Print and shaded views of the part. All mm, measured from the part's lowest x, y and z. A direction names the side the tool comes from. Round coordinates to 2 decimals unless told otherwise and drop trailing zeros. Write each loop counter-clockwise with the first axis right and the second up, starting at its lowest first coordinate (ties: lowest second). Pieces come first, ordered by that corner, then holes. Notation, with made-up numbers: (49, -36.75) -> (64, -36.75) arc R17 cw to (64, -7.75) -> close; hole circle Ø11 at (2.5, 11). An arc over 180 degrees is marked (long way). Return JSON: item names as keys, results as strings. Group by question number.
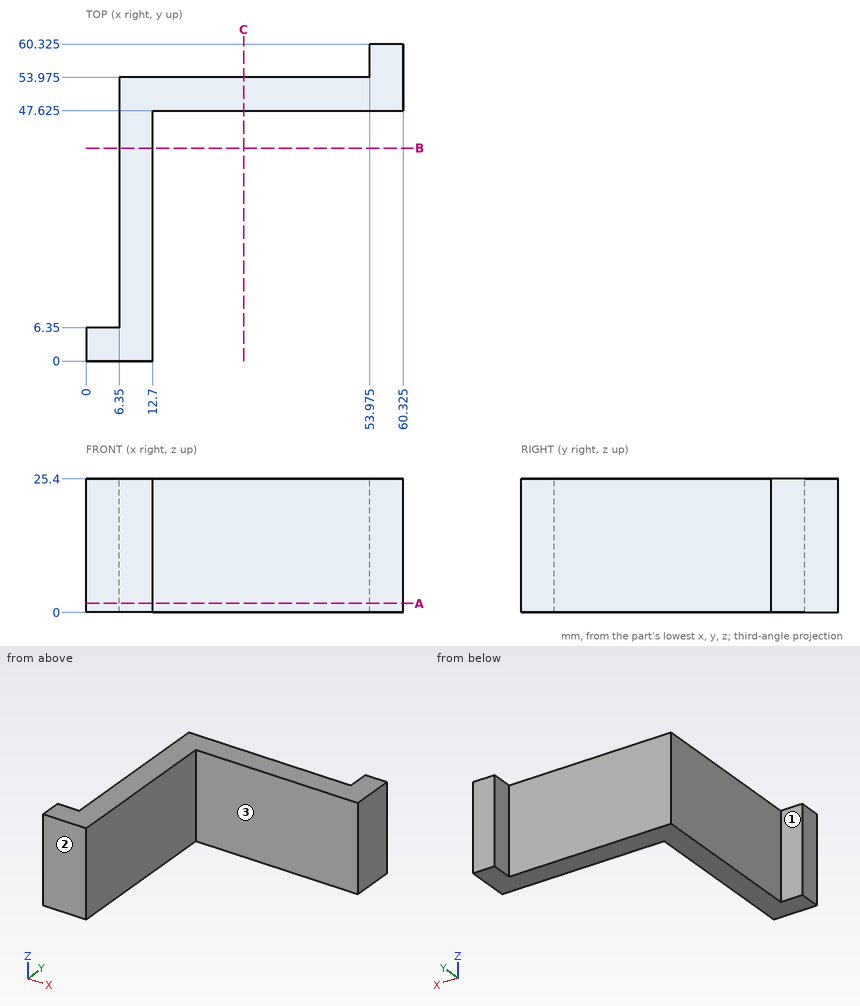
Item 1: Flat gauge pins, fed straight in: P1, Ø2, axis at x = 48, z = 12, coming from the -Y side (3 decimals); P2, Ø5, axis at y = 34.5, z = 13, coming from the -X side; P3, Ø7, axis at x = 4.5, z = 17.5, coming from the +Y side (3 decimals). Where does each tip first touch, or does it go through?
Item 2: Cut at C-C (x = 30). Write the cut outline in (y, z) (3 decimals), then the cut area to 3 significant figures.
Item 3: Cut at A-A (z = 1.75). Write the cut outline in (x, y) (3 decimals).
Item 4: Which spindle directions (+Z, -Z, +X, -X, +Y, -Y) get a long thin tool onto all of the face, cutting with end or side? Do the marked faces 1, 2 and 3. Say none if no direction does.
Item 5: Cut at B-B (y = 40.5). Write the cut outline in (x, z).
Item 6: Wall check: L1, parallel to X at y = 40, z = 20.75; L2, parallel to X at y = 58.5, z = 5.75 (3 decimals); L3, parallel to Y at x = 53.5, z = 6.5 (3 decimals). Give the ranges that are in metal, low to high.
Checks:
{
 "1": {"P1": "stops at y = 47.625", "P2": "stops at x = 6.35", "P3": "stops at y = 53.975"},
 "2": {"outline": "(47.625, 0) -> (53.975, 0) -> (53.975, 25.4) -> (47.625, 25.4) -> close", "area": "161 mm2"},
 "3": {"outline": "(0, 0) -> (12.7, 0) -> (12.7, 47.625) -> (60.325, 47.625) -> (60.325, 60.325) -> (53.975, 60.325) -> (53.975, 53.975) -> (6.35, 53.975) -> (6.35, 6.35) -> (0, 6.35) -> close"},
 "4": {"face 1": "+Z, -Z, -X, +Y", "face 2": "+Z, -Z, +X, -X, -Y", "face 3": "+Z, -Z, +X, -Y"},
 "5": {"outline": "(6.35, 0) -> (12.7, 0) -> (12.7, 25.4) -> (6.35, 25.4) -> close"},
 "6": {"L1": "x = 6.35 to 12.7", "L2": "x = 53.975 to 60.325", "L3": "y = 47.625 to 53.975"}
}
